Source: CAD feature listing. Evaluate the final solid. Frame: model axes, mm. A direction names the side the tool comes from. Give positions to 0.01 mm unless a question says otherwise; leave off trailing zeros. Write each loop counter-clockwise with the first axis right and the second up, starting at its lowest first coordinate (ties: lowest second). Pieces come first, ordered by that corner, then holes. Notation, with made-up numbers: M 21.25,31 L 43.25,31 A21 ccw 43.25,62 Z; hole C 49.5,-34.75 d2. An arc over 180 degrees is marked long. Use CSV: the item, a comma, the result in double quotes. Start each with the question number.
from build123d import *

# Parameters (mm, degrees)
SKETCH1_W               = 90
SKETCH1_H               = 46
SKETCH1_R               = 1.1
BOSS_EXTRUDE1_DEPTH     = 6.35
SKETCH2_W               = 25
SKETCH2_H               = 6.35
BOSS_EXTRUDE2_DEPTH     = 10
FILLET1_R               = 3
MIRROR2_COPY_1_SKETCH_W = 90
MIRROR2_COPY_1_SKETCH_H = 46
MIRROR2_COPY_1_SKETCH_R = 1.1
MIRROR2_COPY_1_DEPTH    = 6.35
FILLET1_OF_MIRROR2_R    = 3
SKETCH3_R               = 2
CUT_EXTRUDE1_DEPTH      = 6.35
SKETCH4_R               = 2
CUT_EXTRUDE2_DEPTH      = 6.35
SKETCH5_R               = 2
CUT_EXTRUDE3_DEPTH      = 6.35
SKETCH6_R               = 2
CUT_EXTRUDE4_DEPTH      = 6.35


with BuildPart() as part:
    # Sketch1 → Boss-Extrude1 (new body)
    with BuildSketch(Plane(origin=(0, 0, 0), x_dir=(1, 0, 0), z_dir=(0, 1, 0))):
        with Locations((45, 23)):
            Rectangle(SKETCH1_W, SKETCH1_H)
        with Locations((85, 5)):
            Circle(SKETCH1_R, mode=Mode.SUBTRACT)
        with Locations((5, 5)):
            Circle(SKETCH1_R, mode=Mode.SUBTRACT)
    boss_extrude1 = extrude(amount=BOSS_EXTRUDE1_DEPTH)

    # Mirror1: Boss-Extrude1 across plane
    add(boss_extrude1.mirror(Plane(origin=(0, 0, -46), x_dir=(1, 0, 0), z_dir=(0, 0, -1))))

    # Sketch2 → Boss-Extrude2 (add)
    with BuildSketch(Plane(origin=(90, 0, 0), x_dir=(0, 0, -1), z_dir=(1, 0, 0))):
        with Locations((12.5, 3.175)):
            Rectangle(SKETCH2_W, SKETCH2_H)
        with Locations((79.5, 3.175)):
            Rectangle(SKETCH2_W, SKETCH2_H)
    boss_extrude2 = extrude(amount=BOSS_EXTRUDE2_DEPTH)

    # Fillet1
    fillet1_edges = [part.edges().sort_by_distance(p)[0] for p in [
        (100, 3.175, 0),
        (100, 3.175, -25),
        (100, 3.175, -92),
        (100, 3.175, -67),
    ]]
    fillet(fillet1_edges, radius=FILLET1_R)

    # Mirror2: Boss-Extrude1, Boss-Extrude2 across plane
    add(boss_extrude1.mirror(Plane(origin=(45, 0, 0), x_dir=(0, 0, 1), z_dir=(1, 0, 0))))
    add(boss_extrude2.mirror(Plane(origin=(45, 0, 0), x_dir=(0, 0, 1), z_dir=(1, 0, 0))))

    # Mirror2 copy 1 sketch → Mirror2 copy 1 (add)
    with BuildSketch(Plane(origin=(90, 0, -92), x_dir=(-1, 0, 0), z_dir=(0, 1, 0))):
        with Locations((45, 23)):
            Rectangle(MIRROR2_COPY_1_SKETCH_W, MIRROR2_COPY_1_SKETCH_H)
        with Locations((85, 5)):
            Circle(MIRROR2_COPY_1_SKETCH_R, mode=Mode.SUBTRACT)
        with Locations((5, 5)):
            Circle(MIRROR2_COPY_1_SKETCH_R, mode=Mode.SUBTRACT)
    extrude(amount=MIRROR2_COPY_1_DEPTH)

    # Fillet1 of Mirror2
    fillet1_of_mirror2_edges = [part.edges().sort_by_distance(p)[0] for p in [
        (-10, 3.175, 0),
        (-10, 3.175, -25),
        (-10, 3.175, -92),
        (-10, 3.175, -67),
    ]]
    fillet(fillet1_of_mirror2_edges, radius=FILLET1_OF_MIRROR2_R)

    # Sketch3 → Cut-Extrude1 (cut)
    with BuildSketch(Plane(origin=(0, 6.35, 0), x_dir=(1, 0, 0), z_dir=(0, 1, 0))):
        with Locations((5, 69)):
            Circle(SKETCH3_R)
        with Locations((85, 69)):
            Circle(SKETCH3_R)
    extrude(amount=-CUT_EXTRUDE1_DEPTH, mode=Mode.SUBTRACT)

    # Sketch4 → Cut-Extrude2 (cut)
    with BuildSketch(Plane(origin=(0, 6.35, 0), x_dir=(1, 0, 0), z_dir=(0, 1, 0))):
        with Locations((5, 23)):
            Circle(SKETCH4_R)
        with Locations((85, 23)):
            Circle(SKETCH4_R)
    extrude(amount=-CUT_EXTRUDE2_DEPTH, mode=Mode.SUBTRACT)

    # Sketch5 → Cut-Extrude3 (cut)
    with BuildSketch(Plane(origin=(0, 6.35, 0), x_dir=(1, 0, 0), z_dir=(0, 1, 0))):
        with Locations((45, 5)):
            Circle(SKETCH5_R)
        with Locations((45, 87)):
            Circle(SKETCH5_R)
    extrude(amount=-CUT_EXTRUDE3_DEPTH, mode=Mode.SUBTRACT)

    # Sketch6 → Cut-Extrude4 (cut)
    with BuildSketch(Plane(origin=(0, 6.35, 0), x_dir=(1, 0, 0), z_dir=(0, 1, 0))):
        with Locations((85, 46)):
            Circle(SKETCH6_R)
        with Locations((45, 46)):
            Circle(SKETCH6_R)
        with Locations((5, 46)):
            Circle(SKETCH6_R)
    extrude(amount=-CUT_EXTRUDE4_DEPTH, mode=Mode.SUBTRACT)


solid = part.part
1. Section B-B on y = 4. Give the number of separate pieces and of enclosed holes in the cut face, then the cut area to 3 significant figures.
2. Line query: probe 1 along Z at (x, y) = (5, 2.5); probe 2 along X at (y, z) = (3.25, -5); probe 3 along X at (y, z) = (1.5, -46). Output: solid intervals per line, ascending.
3. First-contact query: pin 1 (4.5 mm diameter, centred on x = 85, z = -69, fed in from +Y); pin 2 (1.9 mm diameter, centred on y = 3, z = -51.5, fed in from -X). Flat tips, straight axial feed; report the tip coordinate or a pass-through.
4. Section A-A on z = -46. Return loops of the section in (x, y).
5. Access query for faces 5 (the cylindrical face through (86.847, 3.219, -45.234)), 6 (the cylindrical face through (99.14, 3.22, -67.9)), 7 (the cylindrical face through (-9.14, 3.22, -67.9)). Directions: +Z, -Z, +X, -X, +Y, -Y. A direction counts if a zero-diameter tool reaches every point of the face in a straight line with its end or side. Return the directions, or none.
6. Section C-C on z = -30. Return loops of the section in (x, y).
7. Pull-direction query (X, two-part tool) for faces 1 (the cylindrical face through (3.4, 3.2, -21.8)), 2 (the cylindrical face through (99.1, 3.22, -24.14)), 3 (the flat face through (46, 0, -35)), 4 (the cylindrical face through (-9.1, 3.22, -24.14)); classes: released by +X, released by -X, zero draft, split by the parting line, or undercut.
Resolved:
1,separate pieces,"1"
1,enclosed holes,"13"
1,area,"9,140 mm2"
2,probe 1,"z = -92 to -88.1, -85.9 to -71, -67 to -48, -44 to -25, -21 to -6.1, -3.9 to 0"
2,probe 2,"x = -10 to 3.9, 6.1 to 43, 47 to 83.9, 86.1 to 100"
2,probe 3,"x = 0 to 3, 7 to 43, 47 to 83, 87 to 90"
3,pin 1,"stops at y = 6.35"
3,pin 2,"stops at x = 0"
4,outline,"M 0,0 L 3,0 L 3,6.35 L 0,6.35 Z; M 7,0 L 43,0 L 43,6.35 L 7,6.35 Z; M 47,0 L 83,0 L 83,6.35 L 47,6.35 Z; M 87,0 L 90,0 L 90,6.35 L 87,6.35 Z"
5,face 5,"+Y, -Y"
5,face 6,"+X, +Y, -Y"
5,face 7,"-X, +Y, -Y"
6,outline,"M 0,0 L 90,0 L 90,6.35 L 0,6.35 Z"
7,face 1,"undercut"
7,face 2,"released by +X"
7,face 3,"zero draft"
7,face 4,"released by -X"
